from build123d import *

# Parameters (mm, degrees)
SKETCH1_R           = 41
SKETCH1_R_2         = 38
BOSS_EXTRUDE1_DEPTH = 10
SKETCH3_R           = 41
BOSS_EXTRUDE2_DEPTH = 5
SKETCH4_R           = 12.5
BOSS_EXTRUDE3_DEPTH = 5
SKETCH5_R           = 10
CUT_EXTRUDE1_DEPTH  = 6
SKETCH6_R           = 6
CUT_EXTRUDE2_DEPTH  = 5
CUT_EXTRUDE3_DEPTH  = 6


with BuildPart() as part:
    # Sketch1 → Boss-Extrude1 (new body)
    with BuildSketch(Plane(origin=(0, 0, 0), x_dir=(1, 0, 0), z_dir=(0, 1, 0))):
        Circle(SKETCH1_R)
        Circle(SKETCH1_R_2, mode=Mode.SUBTRACT)
    extrude(amount=BOSS_EXTRUDE1_DEPTH)

    # Sketch3 → Boss-Extrude2 (add)
    with BuildSketch(Plane(origin=(0, 10, 0), x_dir=(1, 0, 0), z_dir=(0, 1, 0))):
        Circle(SKETCH3_R)
    extrude(amount=BOSS_EXTRUDE2_DEPTH)

    # Sketch4 → Boss-Extrude3 (add)
    with BuildSketch(Plane.XZ.offset(-10)):
        Circle(SKETCH4_R)
    extrude(amount=BOSS_EXTRUDE3_DEPTH)

    # Sketch5 → Cut-Extrude1 (cut)
    with BuildSketch(Plane.XZ.offset(-5)):
        Circle(SKETCH5_R)
    extrude(amount=-CUT_EXTRUDE1_DEPTH, mode=Mode.SUBTRACT)

    # Sketch6 → Cut-Extrude2 (cut, through all)
    with BuildSketch(Plane.XZ.offset(-11)):
        Circle(SKETCH6_R)
    extrude(amount=-CUT_EXTRUDE2_DEPTH, mode=Mode.SUBTRACT)

    # Sketch7 → Cut-Extrude3 (cut, through all)
    with BuildSketch(Plane.XZ.offset(-10)):
        with BuildLine():
            Line((0, 20), (0, 30))
            ThreePointArc((0, 30), (-15, 25.980762114), (-25.980762114, 15))
            Line((-25.980762114, 15), (-17.320508076, 10))
            ThreePointArc((-17.320508076, 10), (-10, 17.320508076), (0, 20))
        make_face()
        with BuildLine():
            Line((17.320508076, -10), (25.980762114, -15))
            ThreePointArc((25.980762114, -15), (30, 0), (25.980762114, 15))
            Line((25.980762114, 15), (17.320508076, 10))
            ThreePointArc((17.320508076, 10), (20, 0), (17.320508076, -10))
        make_face()
        with BuildLine():
            Line((-17.320508076, -10), (-25.980762114, -15))
            ThreePointArc((-25.980762114, -15), (-15, -25.980762114), (0, -30))
            Line((0, -30), (0, -20))
            ThreePointArc((0, -20), (-10, -17.320508076), (-17.320508076, -10))
        make_face()
    extrude(amount=-CUT_EXTRUDE3_DEPTH, mode=Mode.SUBTRACT)


solid = part.part
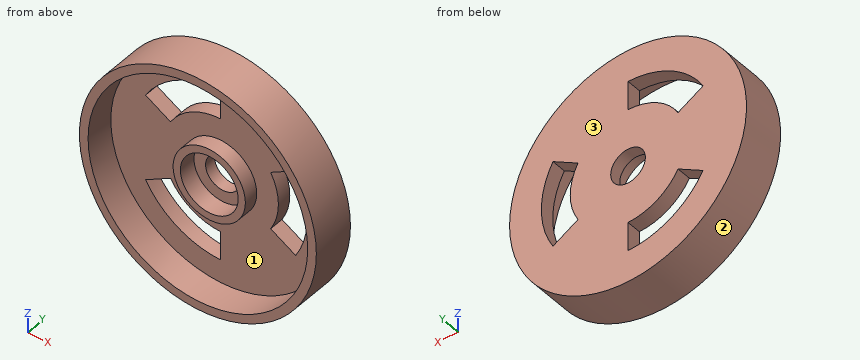
Read the model definition and answer for the solid it produces. Units are mm, in the model's axes. Face numbers are marked on the shaded views. Round coordinates to 2 decimals unless told otherwise and drop trailing zeros. Write each loop counter-clockwise with the first axis right and the second up, starting at its lowest first coordinate (ties: lowest second). Pieces come first, ordered by that corner, then holes.
1. The part is cut by section D-D, the plane y = 6.25. Determine the outline of the cut face in (x, z).
2. Determine the mould class of the marked faces 1, 2 and 3 for opening direction Z: pulls with the +Z half, pulls with the -Z half, needs draft (parallel to the pull), parting line crosses it, or undercut.
3. Given pin 1 Ø6 at (x, z) = (2.5, 3.5) entering from -Y; pin 2 Ø2 at (x, z) = (-23, -5.5) entering from -Y; pin 3 Ø5 at (x, y) = (7.5, 8.5) entering from -Z, each flat-ended and moving along its own axis, determine where each tip first touches the part or whether it passes through.
4. The part is cut by section A-A, the plane z = 0. Determine the outline of the cut face in (x, y), then the cut area to 3 significant figures.
5. Straight lines are drawn through the part: L1, parallel to Z at x = 0, y = 9.2; L2, parallel to Z at x = 6, y = 5.75; L3, parallel to X at y = 2.5, z = 0. For each, find the intervals that lie inside material, in ascending order.
6. The part is cut by section B-B, the plane y = 13.5. Determine the outline of the cut face in (x, z), then the cut area to 3 significant figures.
7. The part is cut by section C-C, the plane z = 28. Determine the outline of the cut face in (x, y).
Values:
1. outline: circle Ø82 at (0, 0); circle Ø25 at (0, 0); hole circle Ø76 at (0, 0); hole circle Ø20 at (0, 0)
2. face 1: undercut
2. face 2: parting line crosses it
2. face 3: needs draft
3. pin 1: stops at y = 11
3. pin 2: stops at y = 10
3. pin 3: stops at z = -40.69
4. outline: (-41, 0) - (-38, 0) - (-38, 10) - (-12.5, 10) - (-12.5, 5) - (-10, 5) - (-10, 11) - (-6, 11) - (-6, 15) - (-41, 15) - close; (6, 11) - (10, 11) - (10, 5) - (12.5, 5) - (12.5, 10) - (20, 10) - (20, 15) - (6, 15) - close; (30, 10) - (38, 10) - (38, 0) - (41, 0) - (41, 15) - (30, 15) - close
4. area: 377 mm2
5. L1: z = -41 to -38, -12.5 to -10, 10 to 12.5, 38 to 41
5. L2: z = -40.56 to -37.52, -10.97 to -8, 8 to 10.97, 37.52 to 40.56
5. L3: x = -41 to -38, 38 to 41
6. outline: circle Ø82 at (0, 0); hole (-25.98, -15) arc R30 ccw to (0, -30) - (0, -20) arc R20 cw to (-17.32, -10) - close; hole (-25.98, 15) - (-17.32, 10) arc R20 cw to (0, 20) - (0, 30) arc R30 ccw to start; hole circle Ø12 at (0, 0); hole (17.32, -10) - (25.98, -15) arc R30 ccw to (25.98, 15) - (17.32, 10) arc R20 cw to start
6. area: 4,380 mm2
7. outline: (-29.95, 0) - (-25.69, 0) - (-25.69, 10) - (-10.77, 10) - (-10.77, 15) - (-29.95, 15) - close; (0, 10) - (25.69, 10) - (25.69, 0) - (29.95, 0) - (29.95, 15) - (0, 15) - close
